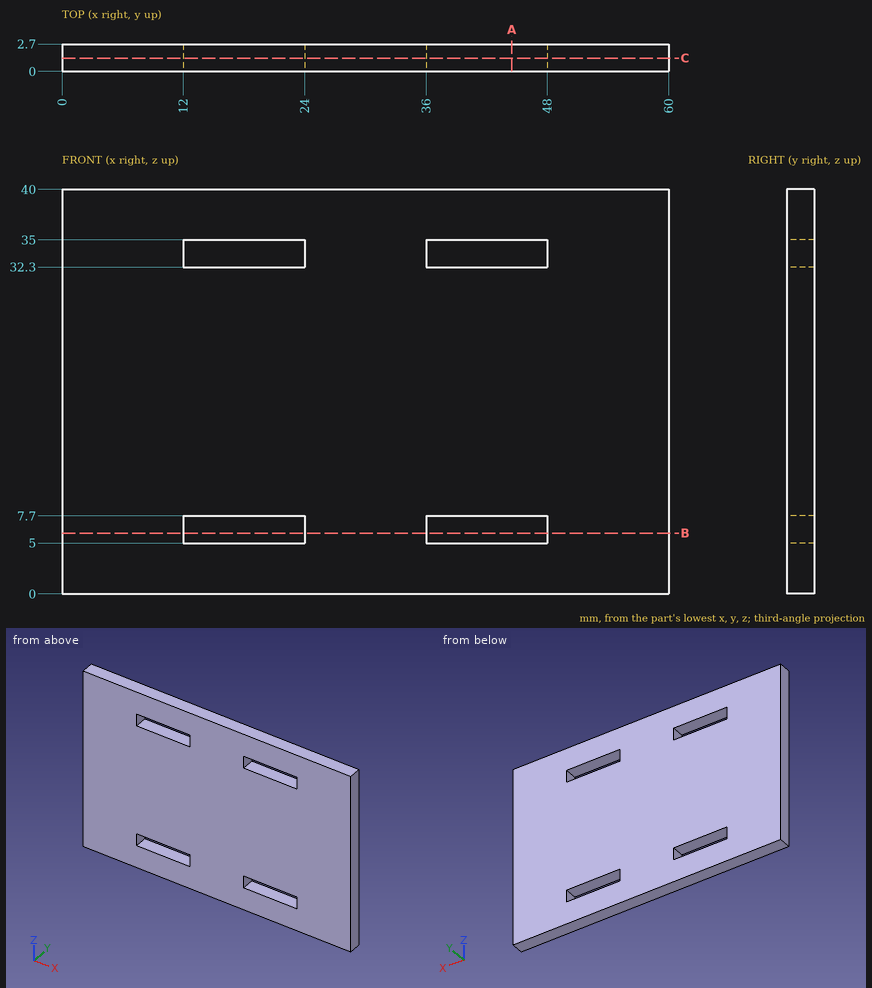
For this review, use the dimensioned drawing (mm, ordinates from the lowest corner) and the shaded views. Give positions to 0.01 mm unless a question says otherwise; leave off trailing zeros. Loops run counter-clockwise (first coordinate to the right, second up) from the corner with the lowest first, then second, coordinate; pieces in that order, holes last.
Item 1: Take a section at A-A, the plane x = 44.5. State the section outline as (y, z) points.
Item 2: Take a section at B-B, the plane z = 6. State the section outline as (x, y) points, and give its area (3 significant figures).
Item 3: For line 1 along Z through (x, y) = (39, 0.4); line 2 along X through (y, z) = (0.7, 7.5), list the stretches that pass through material, from the lowest coordinate up.
Item 4: Take a section at C-C, the plane y = 1.3. State the section outline as (x, z) points, and give its area (3 significant figures).
Calculated:
1. outline: (0, 0) - (2.7, 0) - (2.7, 5) - (0, 5) - close; (0, 7.7) - (2.7, 7.7) - (2.7, 32.3) - (0, 32.3) - close; (0, 35) - (2.7, 35) - (2.7, 40) - (0, 40) - close
2. outline: (0, 0) - (12, 0) - (12, 2.7) - (0, 2.7) - close; (24, 0) - (36, 0) - (36, 2.7) - (24, 2.7) - close; (48, 0) - (60, 0) - (60, 2.7) - (48, 2.7) - close
2. area: 97.2 mm2
3. line 1: z = 0 to 5, 7.7 to 32.3, 35 to 40
3. line 2: x = 0 to 12, 24 to 36, 48 to 60
4. outline: (0, 0) - (60, 0) - (60, 40) - (0, 40) - close; hole (12, 5) - (24, 5) - (24, 7.7) - (12, 7.7) - close; hole (12, 32.3) - (24, 32.3) - (24, 35) - (12, 35) - close; hole (36, 5) - (48, 5) - (48, 7.7) - (36, 7.7) - close; hole (36, 32.3) - (48, 32.3) - (48, 35) - (36, 35) - close
4. area: 2,270 mm2
